```python
from build123d import *

# Parameters (mm, degrees)
F0_W     = 4
F0_H     = 1.8
F0_W_2   = 2
F1_DEPTH = 20
F2_R     = 0.99999


# Not quite as in the source:
# - a fillet or chamfer is up to 0.001 mm smaller than in the source, because OpenCascade refuses the exact size


with BuildPart() as f1:
    # F0 (on Top) → F1 (new body, symmetric)
    with BuildSketch(Plane.XY):
        Polygon((-2, 1.1054119891), (-2, 0.2054119891), (2, 0.2054119891), (4, 0.2054119891), (4, 1.1054119891), align=None)
        with Locations((0, -0.6945880109)):
            Rectangle(F0_W, F0_H)
        with Locations((-3, -0.6945880109)):
            Rectangle(F0_W_2, F0_H)
        with Locations((3, -0.6945880109)):
            Rectangle(F0_W_2, F0_H)
        with Locations((0, -2.4945880109)):
            Rectangle(F0_W, F0_H)
        Polygon((2, -3.3945880109), (-2, -3.3945880109), (-4, -3.3945880109), (-4, -6.3945880109), (29, -6.3945880109), (29, -3.3945880109), (27, -3.3945880109), (23, -3.3945880109), (14.5, -3.3945880109), (10.5, -3.3945880109), align=None)
        with Locations((12.5, -2.4945880109)):
            Rectangle(F0_W, F0_H)
        with Locations((12.5, -0.6945880109)):
            Rectangle(F0_W, F0_H)
        with Locations((9.5, -0.6945880109)):
            Rectangle(F0_W_2, F0_H)
        with Locations((15.5, -0.6945880109)):
            Rectangle(F0_W_2, F0_H)
        with Locations((25, -2.4945880109)):
            Rectangle(F0_W, F0_H)
        Polygon((8.5, 0.2054119891), (10.5, 0.2054119891), (14.5, 0.2054119891), (16.5, 0.2054119891), (16.5, 1.1054119891), (8.5, 1.1054119891), align=None)
        with Locations((25, -0.6945880109)):
            Rectangle(F0_W, F0_H)
        with Locations((22, -0.6945880109)):
            Rectangle(F0_W_2, F0_H)
        with Locations((28, -0.6945880109)):
            Rectangle(F0_W_2, F0_H)
        Polygon((21, 0.2054119891), (23, 0.2054119891), (27, 0.2054119891), (27, 1.1054119891), (21, 1.1054119891), align=None)
    extrude(amount=F1_DEPTH, both=True)

    # F2 (radius 1 in the source; OpenCascade refuses exactly that, so slightly less here)
    f2_edges = [f1.edges().sort_by_distance(p)[0] for p in [
        (-2, -1.594588, 0),
        (2, -1.594588, 0),
        (10.5, -1.594588, 0),
        (14.5, -1.594588, 0),
        (23, -1.594588, 0),
        (27, -1.594588, 0),
        (8.5, -1.594588, 0),
        (-4, -1.594588, 0),
        (21, -1.594588, 0),
        (16.5, -1.594588, 0),
        (29, -1.594588, 0),
        (4, -1.594588, 0),
    ]]
    fillet(f2_edges, radius=F2_R)


solid = f1.part
```
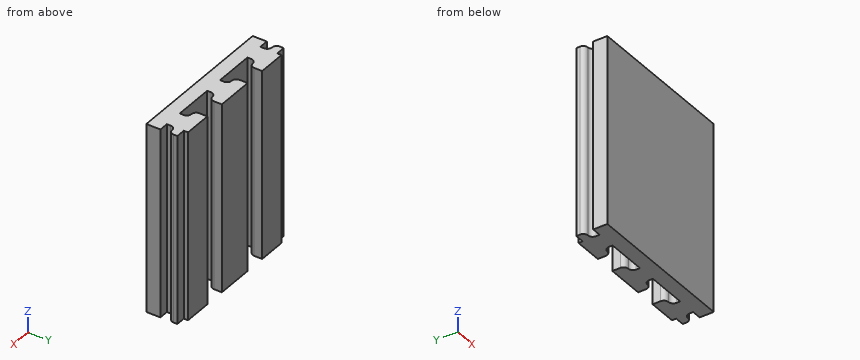
Build history of the part. All positions in model axes, mm. Give positions to 0.01 mm unless a question says otherwise; leave off trailing zeros. Loops run counter-clockwise (first coordinate to the right, second up) from the corner with the lowest first, then second, coordinate; pieces in that order, holes last.
1) Drop flat-ended pins along their axis: P1, Ø0.5, axis at y = 0.5, z = 2.5, coming from the -X side; P2, Ø1, axis at x = 28, z = 2.5, coming from the +Y side. Give the stop position or say it passes through.
Values follow:
P1: stops at x = -2
P2: stops at y = 0.21
2) Band-saw the part on B-B on x = 17.5. List the corners of the cut face in (y, z).
Values follow:
outline: (-6.39, -20) - (-3.39, -20) - (-3.39, 20) - (-6.39, 20) - close
3) Band-saw the part on A-A on x = 10. List the corners of the cut face in (y, z), then the cut area to 3 significant figures.
Values follow:
outline: (-6.39, -20) - (-3.39, -20) - (-3.39, 20) - (-6.39, 20) - close; (-1.73, -20) - (1.11, -20) - (1.11, 20) - (-1.73, 20) - close
area: 233 mm2
4) Probe line 1 along X through (y, z) = (0, 5); line 2 along X through (y, z) = (0.5, -17); line 3 along Y through (x, z) = (8, -17). List the from-to ranges inside material, lowest first.
Values follow:
line 1: x = -4 to 4, 8.5 to 16.5, 21 to 29
line 2: x = -2 to 4, 8.5 to 16.5, 21 to 27
line 3: y = -6.39 to -3.39
